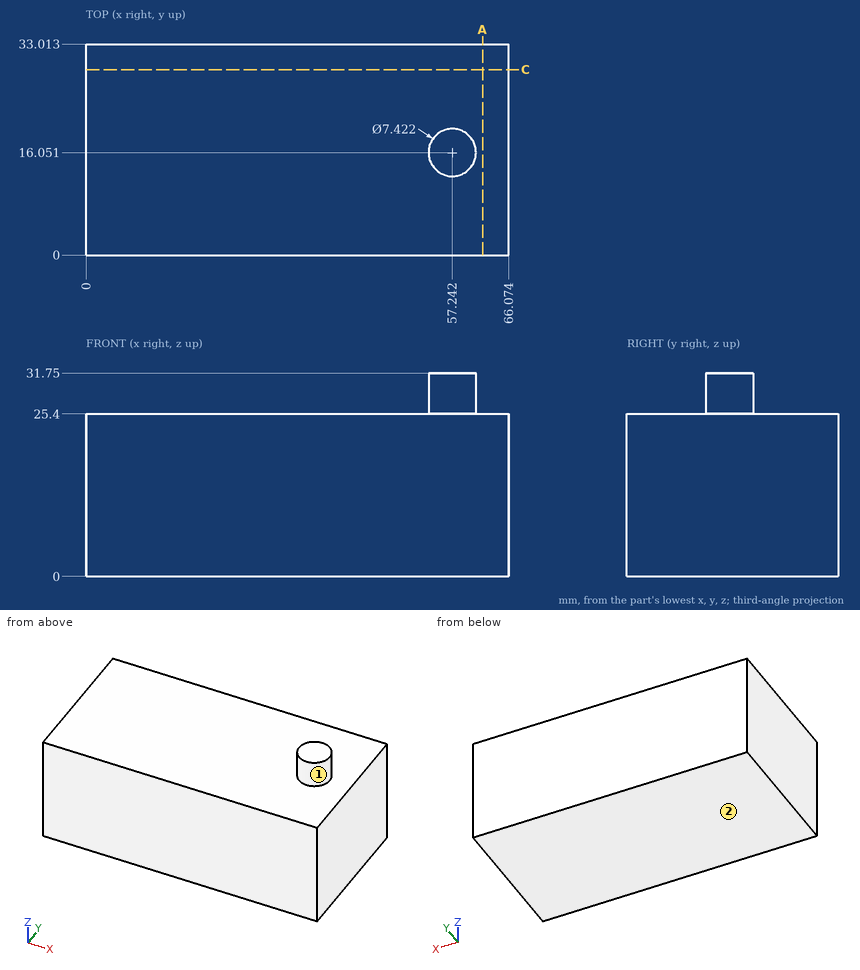
Answer from the drawing. Dimensions are ordinates in mm from the lowest x, y and z of the part. A direction names the side the tool comes from. Coordinates: 2 decimals unless noted, no trailing zeros. Loops run counter-clockwise (first coordinate to the right, second up) from the corner with the lowest first, then second, coordinate; pieces in that order, holes last. Notation, with made-up numbers: (86.5, 31) -> (97.5, 31) arc R26 ccw to (97.5, 63) -> close; hole circle Ø2 at (44, 64). An arc over 180 degrees is marked (long way). Return JSON: item names as keys, results as strings.
Item 1: Find section A-A (x = 62). Determine the outline of the cut face in (y, z).
Answers:
{"outline": "(0, 0) -> (33.01, 0) -> (33.01, 25.4) -> (0, 25.4) -> close"}
Item 2: Find section C-C (y = 29). Determine the outline of the cut face in (x, z) (1 decimal).
Answers:
{"outline": "(0, 0) -> (66.1, 0) -> (66.1, 25.4) -> (0, 25.4) -> close"}
Item 3: Find the intervals of material crossed by probe 1 along Z at (x, y) = (48, 15), in increasing order.
Answers:
{"probe 1": "z = 0 to 25.4"}
Item 4: For the marked faces 1 and 2, determine the directions among +Z, -Z, +X, -X, +Y, -Y from which every point of the face is accessible in a straight line to the end or side of a thin tool.
Answers:
{"face 1": "+Z", "face 2": "-Z, +X, -X, +Y, -Y"}
Item 5: A flat-ended cylindrical pin translates along its axis: P1, Ø16.5, axis at x = 18.5, y = 20, coming from the +Z side. Find the tip coordinate at first contact, or state that the pin passes through.
Answers:
{"P1": "stops at z = 25.4"}
